```python
from build123d import *

# Parameters (mm, degrees)
SKETCH1_R           = 2
BOSS_EXTRUDE1_DEPTH = 4
SKETCH2_R           = 2
BOSS_EXTRUDE2_DEPTH = 2


with BuildPart() as part:
    # Sketch1 → Boss-Extrude1 (new body)
    with BuildSketch(Plane(origin=(0, 0, 0), x_dir=(1, 0, 0), z_dir=(0, 1, 0))):
        with BuildLine():
            Line((2.12569774, -5.610829628), (14.125697613, -1.064554922))
            ThreePointArc((14.125697613, -1.064554922), (17.99688746, 4.353037094), (14.482508262, 10.008614247))
            Line((14.482508262, 10.008614247), (2.482508267, 15.46233949))
            ThreePointArc((2.482508267, 15.46233949), (-3.248457357, 15.044553975), (-6, 10))
            Line((-6, 10), (-6, 0))
            ThreePointArc((-6, 0), (-3.409238446, -4.937316398), (2.12569774, -5.610829628))
        make_face()
        with Locations(Location((0, 0, 0), (0, 0, 270))):
            Circle(SKETCH1_R, mode=Mode.SUBTRACT)
        with Locations(Location((0, 10, 0), (0, 0, 270))):
            Circle(SKETCH1_R, mode=Mode.SUBTRACT)
        with Locations(Location((12, 4.546274754, 0), (0, 0, 270))):
            Circle(SKETCH1_R, mode=Mode.SUBTRACT)
    extrude(amount=BOSS_EXTRUDE1_DEPTH)

    # Sketch2 → Boss-Extrude2 (add)
    with BuildSketch(Plane(origin=(0, 4, 0), x_dir=(1, 0, 0), z_dir=(0, 1, 0))):
        with BuildLine():
            ThreePointArc((6, 10), (0, 16), (-6, 10))
            Line((-6, 10), (-6, 0))
            ThreePointArc((-6, 0), (0, -6), (6, 0))
            Line((6, 0), (6, 10))
        make_face()
        Circle(SKETCH2_R, mode=Mode.SUBTRACT)
        with Locations((0, 10)):
            Circle(SKETCH2_R, mode=Mode.SUBTRACT)
    extrude(amount=BOSS_EXTRUDE2_DEPTH)


solid = part.part
```
The listing builds one solid part. Answer for the finished solid, in the listing's coordinates (mm). A direction names the side the tool comes from. Coordinates: 2 decimals unless noted, no trailing zeros. Write each loop counter-clockwise with the first axis right and the second up, starting at its lowest first coordinate (ties: lowest second). Pieces come first, ordered by that corner, then holes. Notation, with made-up numbers: (68, 5) - (74, 5) arc R25 cw to (74, 35) - close; hole circle Ø9 at (28, 10). An arc over 180 degrees is marked (long way). Return JSON: item names as keys, results as strings. Group by question number.
1. Determine the mould class of faces 3 (the flat face through (0, 6, -5)), 4 (the cylindrical face through (13.35, 1.97, -6.02)), 5 (the flat face through (-6, 3, -5)) for opening direction X: released by +X, released by -X, zero draft, split by the parting line, or undercut.
2. Straight lines are drawn through the part: L1, parallel to Z at x = 0, y = 1.7; L2, parallel to X at y = 4.85, z = 0; L3, parallel to Y at x = 8.25, z = -12.5. For each, find the intervals that lie inside material, in ascending order.
3. A cutting plane is placed at D-D, the plane z = 3.75. Determine the outline of the cut face in (x, y), plus the area to 3 significant figures.
4. A cutting plane is placed at C-C, the plane x = 12. Determine the outline of the cut face in (y, z), plus the area to 3 significant figures.
5. Given pin 1 (1 mm diameter, centred on y = 5.5, z = -3.5, fed in from +X); pin 2 (1.5 mm diameter, centred on x = 10, z = 1, fed in from +Y); pin 3 (1.5 mm diameter, centred on x = 5, y = 4.5, fed in from +Z), each flat-ended and moving along its own axis, determine where each tip first touches the part or whether it passes through.
6. A cutting plane is placed at B-B, the plane y = 2.4. Determine the outline of the cut face in (x, z), plus the area to 3 significant figures.
7. Which of the six approach directions +Z, -Z, +X, -X, +Y, -Y give full straight-line access (tool end or side, diameter ignored) to faces 1 (the flat face through (6, 5, -5)), 2 (the cylindrical face through (17.993, 1.972, -4.254))?
8. A cutting plane is placed at A-A, the plane z = -0.5. Determine the outline of the cut face in (x, y), plus the area to 3 significant figures.
Ans:
{
 "1": {"face 3": "zero draft", "face 4": "undercut", "face 5": "released by -X"},
 "2": {"L1": "-16 to -12, -8 to -2, 2 to 6", "L2": "-6 to -2, 2 to 6", "L3": "0 to 4"},
 "3": {"outline": "(-4.68, 0) - (7.04, 0) - (7.04, 4) - (4.68, 4) - (4.68, 6) - (-4.68, 6) - close", "area": "65.6 mm²"},
 "4": {"outline": "(0, -11.14) - (4, -11.14) - (4, -6.55) - (0, -6.55) - close; (0, -2.55) - (4, -2.55) - (4, 1.87) - (0, 1.87) - close", "area": "36.0 mm²"},
 "5": {"pin 1": "x = 6", "pin 2": "y = 4", "pin 3": "z = 4.73"},
 "6": {"outline": "(-6, -10) arc R6 ccw to (2.48, -15.46) - (14.48, -10.01) arc R6 ccw to (14.13, 1.06) - (2.13, 5.61) arc R6 ccw to (-6, 0) - close; hole circle Ø4 at (0, -10); hole circle Ø4 at (0, 0); hole circle Ø4 at (12, -4.55)", "area": "351 mm²"},
 "7": {"face 1": "+Z, -Z, +X, +Y", "face 2": "+X, +Y, -Y"},
 "8": {"outline": "(-6, 0) - (-1.94, 0) - (-1.94, 6) - (-6, 6) - close; (1.94, 0) - (16.43, 0) - (16.43, 4) - (6, 4) - (6, 6) - (1.94, 6) - close", "area": "90.5 mm²"}
}
